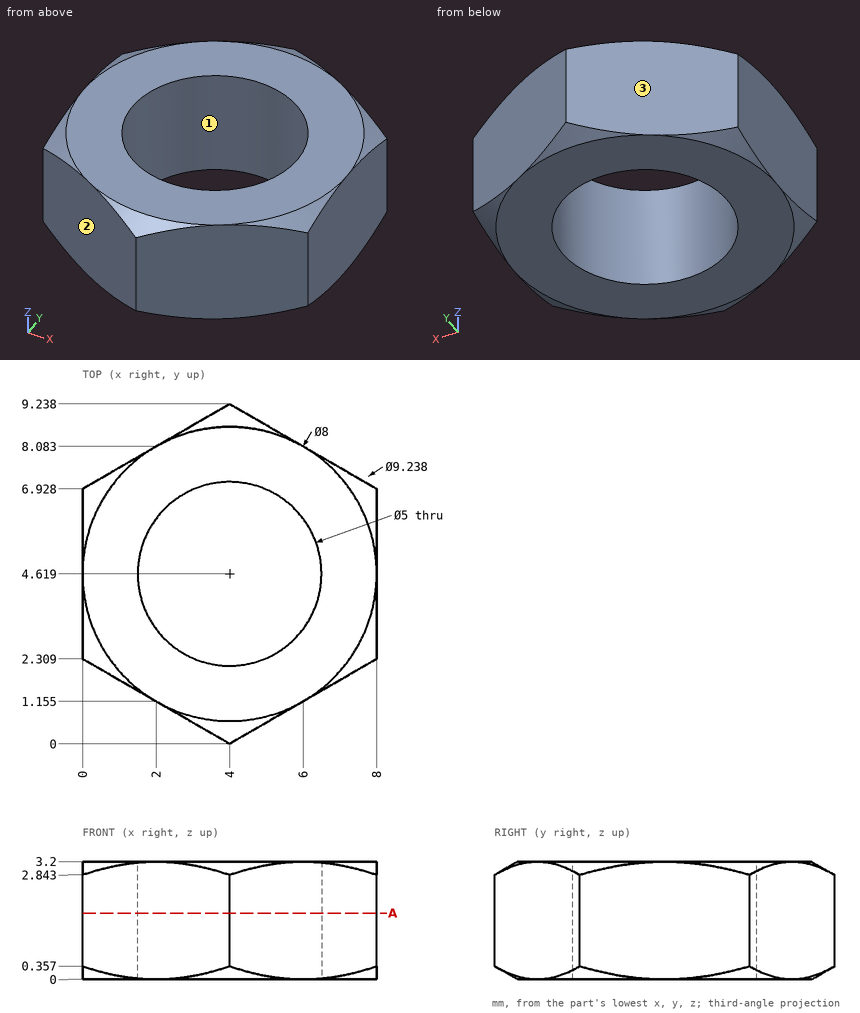
Geometry: see drawing. Coordinates: mm, zero at the bounding-box minimum. Round coordinates to 2 decimals unless told otherwise and drop trailing zeros. Order: outer loops, then holes, each group sorted by start corner. A loop starts at its lowest first (then second) coordinate and runs counter-clockwise, first axis right, second up. Notation, with made-up numbers: (-19, 9.25) - (23, 9.25) arc R36 cw to (23, 45.25) - close; hole circle Ø10 at (-9, 29). An arc over 180 degrees is marked (long way). Use a Markdown table: item, result. Add a question column.
1. Line query: probe 1 along X at (y, z) = (4.5, 2.1); probe 2 along Y at (x, z) = (3.25, 2.5) (1 decimal); probe 3 along X at (y, z) = (5.25, 1.6). Output: solid intervals per line, ascending.
2. First-contact query: pin 1 (3 mm diameter, centred on x = 2.5, y = 6, fed in from +Z); pin 2 (1.5 mm diameter, centred on x = 1, z = 1.5, fed in from +Y). Flat tips, straight axial feed; report the tip coordinate or a pass-through.
3. Mould query, pull axis Y, two halves, no side actions, for the marked faces 1, 2 and 3. Classes: +Y half, -Y half, draft (parallel to the pull), parting line (faces both ways), or undercut.
4. Section query A-A (z = 1.8). Return the cut outline in (x, y), then the cut area to 3 significant figures.
Derived:
| question | item | result |
|---|---|---|
| 1 | probe 1 | 0 to 1.5, 6.5 to 8 |
| 1 | probe 2 | 0.4 to 2.2, 7 to 8.8 |
| 1 | probe 3 | 0 to 1.58, 6.42 to 8 |
| 2 | pin 1 | z = 3.2 |
| 2 | pin 2 | y = 7.94 |
| 3 | face 1 | undercut |
| 3 | face 2 | -Y half |
| 3 | face 3 | +Y half |
| 4 | outline | (0, 2.31) - (4, 0) - (8, 2.31) - (8, 6.93) - (4, 9.24) - (0, 6.93) - close; hole circle Ø5 at (4, 4.62) |
| 4 | area | 35.8 mm2 |
